For this review, take the finished solid that the model builds, in its own axes (mm). Face numbers are marked on the shaded views. A direction names the side the tool comes from. Give positions to 0.01 mm unless a question says otherwise; leave off trailing zeros. Order: outer loops, then holes, each group sorted by start corner. A loop starts at its lowest first (then second) coordinate and runs counter-clockwise, first axis right, second up. Notation, with made-up numbers: (32, 7) -> (36, 7) arc R21 ccw to (36, 13) -> close; hole circle Ø4 at (15.25, 66.5). An arc over 180 degrees is marked (long way). Return JSON: item names as keys, results as strings. Group by question number.
1) Add section B-B (x = -16). Give the boundary of the cut face in (y, z), then the cut area to 3 significant figures.
2) Insertion check: P1, Ø3, axis at x = 16, y = -15, coming from the -Z side; P2, Ø8, axis at x = -13, z = -7, coming from the +Y side; P3, Ø3, axis at x = -13.5, y = -10.5, coming from the +Z side; P4, Ø2, axis at y = -5.5, z = 11, coming from the -X side. Each pin has a flat end and moves straight along its axis. Give the tip position at first contact, or say it passes through.
3) To check wall thickness, follow line 1 along Y through (x, z) = (16, 7.55); line 2 along Z through (x, y) = (-8.5, 13); line 3 along Z through (x, y) = (8, -1). State the ranges of each line that lie inside material, in increasing order.
4) For the marked faces 1, 2, 3, 4 and 5, list the 3-axis set-ups (+Z, -Z, +X, -X, +Y, -Y) from which the entire face can be reached by the end or side of a thin tool; tool diameter is ignored.
5) Add section A-A (y = -15). State how many separate pieces and enclosed holes the cut face has, then the cut area to 3 significant figures.
6) Add section C-C (y = 4). Give the boundary of the cut face in (x, z), then the cut area to 3 significant figures.
7) The part is to be moulded in two halves that separate along X. For the marked faces 6, 7 and 8, say which applies: released by +X, released by -X, zero draft, split by the parting line, or undercut.
8) Add section D-D (x = 16). Give the boundary of the cut face in (y, z), then the cut area to 3 significant figures.
from build123d import *

# Parameters (mm, degrees)
F1_DEPTH = 25
F3_D     = 6.7564
F4_W     = 69.7505115181
F4_H     = 20
F5_DEPTH = 40.001
F7_DEPTH = 10
F9_D     = 5.1054


# Not quite as in the source:
# - a feature names something its author has since deleted; it is built from what else it names


with BuildPart() as f1:
    # F0 (on Front) → F1 (new body, symmetric)
    with BuildSketch(Plane.XZ):
        Polygon((10, 27), (0, 27), (0, 15), (-10, 15), (-10, 8.5), (-20, 8.5), (-20, -1.5), (-10, -1.5), (-10, -20), (10, -20), (10, -1.5), (20, -1.5), (20, 8.5), (10, 8.5), align=None)
    extrude(amount=F1_DEPTH, both=True)

    # F3 (through all)
    with Locations(Plane.XZ.offset(25)):
        with Locations((0, 0)):
            Hole(F3_D / 2)

    # F4 (on face) → F5 (cut, through all)
    with BuildSketch(Plane.YZ.offset(20)):
        with Locations((29.875255759, 0)):
            Rectangle(F4_W, F4_H)
    extrude(amount=-F5_DEPTH, mode=Mode.SUBTRACT)

    # F6 (on face) → F7 (cut)
    with BuildSketch(Plane.YZ.offset(20)):
        with BuildLine():
            ThreePointArc((-20, 7), (-23.5, 3.5), (-20, 0))
            Line((-20, 0), (-5, 0))
            Line((-5, 0), (-5, 7))
            Line((-5, 7), (-20, 7))
        make_face()
    extrude(amount=-F7_DEPTH, mode=Mode.SUBTRACT)

    # F9 (through all)
    with Locations(Plane.XY.offset(8.5)):
        with Locations((16, -15), (-16, -15)):
            Hole(F9_D / 2)


solid = f1.part
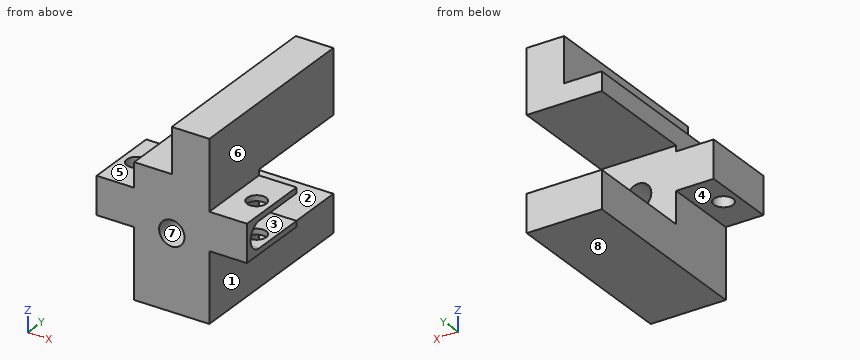
Evaluation:
{
 "1": {"outline": "(-25, -1.5) -> (-17.55, -1.5) -> (-17.55, 8.5) -> (-25, 8.5) -> close; (-12.45, -1.5) -> (-5, -1.5) -> (-5, 8.5) -> (-12.45, 8.5) -> close", "area": "149 mm^2"},
 "2": {"P1": "through", "P2": "y = -5", "P3": "z = 8.5", "P4": "x = -10"},
 "3": {"line 1": "-25 to -17.55, -12.45 to -5", "line 2": "-20 to -10, 10 to 15", "line 3": "-20 to -10, 10 to 27"},
 "4": {"face 1": "-Z, +X, +Y, -Y", "face 2": "+X, -X, +Y", "face 3": "+X, +Y", "face 4": "-Z, -X, +Y, -Y", "face 5": "+Z, -X, +Y, -Y"},
 "5": {"separate pieces": "4", "enclosed holes": "1", "area": "848 mm^2"},
 "6": {"outline": "(-10, -20) -> (10, -20) -> (10, -10) -> (-10, -10) -> close; (-10, 10) -> (10, 10) -> (10, 27) -> (0, 27) -> (0, 15) -> (-10, 15) -> close", "area": "420 mm^2"},
 "7": {"face 6": "released by +X", "face 7": "undercut", "face 8": "zero draft"},
 "8": {"outline": "(-25, -1.5) -> (-17.55, -1.5) -> (-17.55, 0) -> (-20, 0) arc R3.5 cw to (-20, 7) -> (-17.55, 7) -> (-17.55, 8.5) -> (-25, 8.5) -> close; (-12.45, -1.5) -> (-5, -1.5) -> (-5, 0) -> (-12.45, 0) -> close; (-12.45, 7) -> (-5, 7) -> (-5, 8.5) -> (-12.45, 8.5) -> close", "area": "60.4 mm^2"}
}
